Design review of the part built by this model. Coordinates are the model's own, in mm. Face numbers are marked on the shaded views. A direction names the side the tool comes from. Give positions to 0.01 mm unless a question says otherwise; leave off trailing zeros. Loops run counter-clockwise (first coordinate to the right, second up) from the corner with the lowest first, then second, coordinate; pieces in that order, holes last. Notation, with made-up numbers: (-27, 40) - (25, 40) arc R22 ccw to (25, 74) - close; hole circle Ø9 at (30.25, 62). An arc over 180 degrees is marked (long way). Write each question's results on one line, items separated by ' | '.
Autodesk Fusion 360 part; units mm, degrees
sketch "スケッチ1" plane through (0, 0, 0) normal (0, 0, 1) x (1, 0, 0)
  circle A0 centre (0, 0) radius 11
  dimension "d1" = 22
extrude "押し出し1" add sketch "スケッチ1" along normal blind 18
sketch "スケッチ2" plane through (0, 0, 18) normal (0, 0, 1) x (1, 0, 0)
  circle A0 centre (0, 0) radius 11
  circle A1 centre (0, 0) radius 10
  line L0 (-7, -7.7) -> (7, -7.7)
  line L1 (7, -7.7) -> (7, 7.7)
  line L2 (7, 7.7) -> (-7, 7.7)
  line L3 (-7, 7.7) -> (-7, -7.7)
  line L4 (-7, -7.7) -> (7, 7.7) construction
  line L5 (7, -7.7) -> (-7, 7.7) construction
  dimension "d4" = 20
  dimension "d5" = 14
  dimension "d6" = 15.4
sketch "スケッチ3" plane through (0, 0, 18) normal (0, 0, 1) x (1, 0, 0)
extrude "押し出し2" add sketch "スケッチ2" along normal blind 32 contours A1 L1 | A1 L0 L1 L2 L3 | A1 L3
sketch "スケッチ4" plane through (0, 0, 50) normal (0, 0, 1) x (1, 0, 0)
  arc A0 (6.3804, -7.7) -> (6.3804, 7.7) centre (0, 0) ccw
  line L0 (6.3804, 7.7) -> (-6.3804, 7.7)
  arc A1 (-6.3804, 7.7) -> (-6.3804, -7.7) centre (0, 0) ccw
  line L1 (-6.3804, -7.7) -> (6.3804, -7.7)
  circle A2 centre (0, 0) radius 10.2
  dimension "d9" = 20.4
extrude "押し出し3" add sketch "スケッチ4" along normal blind 9 contours A0 L0 A1 L1 | A2
sketch "スケッチ5" plane through (0, 0, 0) normal (0, 0, -1) x (-1, 0, 0)
  circle A0 centre (0, 0) radius 11
  circle A1 centre (0, 0) radius 6.9
  line L0 (6, 3.45) -> (-6, 3.45)
  line L1 (-6, 3.45) -> (-6, -3.45)
  line L2 (-6, -3.45) -> (6, -3.45)
  line L3 (6, -3.45) -> (6, 3.45)
  line L4 (6, 3.45) -> (-6, -3.45) construction
  line L5 (-6, 3.45) -> (6, -3.45) construction
  dimension "d12" = 13.8
  dimension "d13" = 12
  dimension "d14" = 6.9
extrude "押し出し4" add sketch "スケッチ5" along normal blind 2 contours A1 L3 | A1 L0 L1 L2 L3 | A1 L1
sketch "スケッチ6" plane through (0, 0, -2) normal (0, 0, -1) x (-1, 0, 0)
  arc A0 (-5.9756, 3.45) -> (-5.9756, -3.45) centre (0, 0) ccw
  line L0 (-5.9756, -3.45) -> (5.9756, -3.45)
  arc A1 (5.9756, -3.45) -> (5.9756, 3.45) centre (0, 0) ccw
  line L1 (5.9756, 3.45) -> (-5.9756, 3.45)
  circle A2 centre (0, 0) radius 2
  dimension "d17" = 4
extrude "押し出し5" add sketch "スケッチ6" along normal blind 4 contours A2
sketch "スケッチ8" plane through (0, 0, 18) normal (0, 0, 1) x (1, 0, 0)
  circle A0 centre (0, 0) radius 2
  dimension "d22" = 4
extrude "押し出し6" add 1 faces at (-0.637, 0.1965, -6) along direction (0, 0, -1) blind 8
sketch "スケッチ9" plane through (0, 0, -14) normal (0, 0, -1) x (-1, 0, 0)
  circle A0 centre (0, 0) radius 2
  line L0 (0, 2) -> (-2.3, 2)
  line L1 (-2.3, 2) -> (-2.3, 1.5)
  line L2 (-2.3, 1.5) -> (0, 1.5)
  line L3 (0, 1.5) -> (0, 2)
  circle A1 centre (0, 0) radius 2
  line L4 (0, 1.5) -> (1.7491, 1.5)
  line L5 (1.7491, 1.5) -> (1.7491, 2)
  line L6 (1.7491, 2) -> (0, 2)
  line L7 (0, 2) -> (0, 1.5)
extrude "押し出し7" cut sketch "スケッチ9" against normal blind 8 contours A0 L3 A1 L4 L7 | A0 L2 L3 A1 L7
sketch "スケッチ10" plane through (0, 0, 0) normal (0, 0, -1) x (-1, 0, 0)
  line L0 (-5.9756, 3.45) -> (5.9756, 3.45)
  arc A0 (5.9756, -3.45) -> (5.9756, 3.45) centre (0, 0) ccw
  line L1 (5.9756, -3.45) -> (-5.9756, -3.45)
  arc A1 (-5.9756, 3.45) -> (-5.9756, -3.45) centre (0, 0) ccw
  circle A2 centre (0, 0) radius 11
  circle A3 centre (0, 0) radius 7
  line L2 (7, 6) -> (-7, 6)
  line L3 (-7, 6) -> (-7, -6)
  line L4 (-7, -6) -> (7, -6)
  line L5 (7, -6) -> (7, 6)
  line L6 (7, 6) -> (-7, -6) construction
  line L7 (-7, 6) -> (7, -6) construction
  dimension "d27" = 14
  dimension "d28" = 14
  dimension "d29" = 12
extrude "押し出し8" add sketch "スケッチ10" along normal blind 2 contours A3 L2 L4
sketch "スケッチ11" plane through (0, 0, 0) normal (0, 0, -1) x (-1, 0, 0)
  line L0 (-3.6056, 6) -> (3.6056, 6)
  arc A0 (3.6056, -6) -> (3.6056, 6) centre (0, 0) ccw
  line L1 (3.6056, -6) -> (-3.6056, -6)
  arc A1 (-3.6056, 6) -> (-3.6056, -6) centre (0, 0) ccw
  circle A2 centre (0, 0) radius 11
sketch "スケッチ12" plane through (0, 0, 0) normal (0, 0, -1) x (-1, 0, 0)
  line L0 (11, 0) -> (-11, 0)
  line L1 (-11, 0) -> (-11, -11)
  line L2 (-11, -11) -> (0, 0)
  line L3 (0, 0) -> (7.7782, 7.7782)
  circle A0 centre (0, 0) radius 9
  circle A1 centre (-6.364, -6.364) radius 1
  line L4 (0, 1.75) -> (0, 22.5)
  circle A2 centre (6.364, -6.364) radius 1
  circle A3 centre (6.364, 6.364) radius 1
  circle A4 centre (-6.364, 6.364) radius 1
  dimension "d32" = 11
  dimension "d33" = 180
  dimension "d34" = 11
  dimension "d35" = 18
  dimension "d36" = 2
extrude "押し出し9" cut sketch "スケッチ12" against normal blind 4 contours L3 A0 A3 | L3 A0 A3 | A0 A2 | A0 A2 | L2 A0 A1 | L2 A0 A1 | L3 A0 A3 | L3 A0 A3 | A0 A4 | A0 A4 | L2 A0 A1 | L2 A0 A1
sketch "スケッチ14" plane through (0, 0, 50) normal (0, 0, -1) x (-1, 0, 0)
  circle A0 centre (0, 0) radius 10.2
  line L0 (6.3804, -7.7) -> (-6.3804, -7.7)
  arc A1 (-6.3804, 7.7) -> (-6.3804, -7.7) centre (0, 0) ccw
  line L1 (-6.3804, 7.7) -> (6.3804, 7.7)
  arc A2 (6.3804, -7.7) -> (6.3804, 7.7) centre (0, 0) ccw
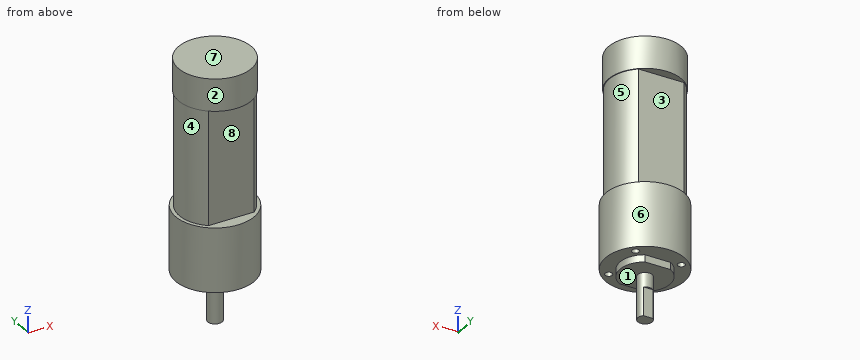
Item 1: We need section D-D on y = 4. Give the boundary of the cut face in (x, z), then the cut area to 3 significant figures.
Output values:
outline: (-10.25, 0) - (-5.74, 0) - (-5.74, -2) - (5.74, -2) - (5.74, 0) - (10.25, 0) - (10.25, 18) - (9.17, 18) - (9.17, 50) - (9.38, 50) - (9.38, 59) - (-9.38, 59) - (-9.38, 50) - (-9.17, 50) - (-9.17, 18) - (-10.25, 18) - close | area: 1,150 mm²
Item 2: Clearance check with flat-ended pins moving along their axes: P1, Ø6, axis at x = -2, y = 4, coming from the -Z side; P2, Ø0.6, axis at x = -1, z = -1.5, coming from the -Y side; P3, Ø1, axis at x = -7, y = -6.5, coming from the -Z side; P4, Ø10, axis at y = -8.5, z = 6.5, coming from the -X side. State where each tip first meets the part, or that it passes through.
Output values:
P1: stops at z = -14 | P2: stops at y = -6 | P3: stops at z = 0 | P4: stops at x = -10.43
Item 3: Tool access review of the marked faces 1, 2, 3 and 4: name each direction out of +Z, -Z, +X, -X, +Y, -Y from which nothing blocks a thin tool from reaching the whole face with its end or side.
Output values:
face 1: -Z | face 2: +Z | face 3: +X, -X, +Y | face 4: -X
Item 4: Draft analysis for pull direction Z (two halves, no side actions). For the marked faces 5, 6, 7 and 8, state which applies: +Z half, -Z half, draft (parallel to the pull), parting line (faces both ways), or undercut.
Output values:
face 5: undercut | face 6: draft | face 7: +Z half | face 8: undercut
Item 5: We need section A-A on x = 0. Give the boundary of the cut face in (y, z), then the cut area to 3 significant figures.
Output values:
outline: (-11, 0) - (-6, 0) - (-6, -2) - (-2, -2) - (-2, -14) - (1.5, -14) - (1.5, -6) - (2, -6) - (2, -2) - (6, -2) - (6, 0) - (11, 0) - (11, 18) - (7.7, 18) - (7.7, 50) - (10.2, 50) - (10.2, 59) - (-10.2, 59) - (-10.2, 50) - (-7.7, 50) - (-7.7, 18) - (-11, 18) - close | area: 1,140 mm²
Item 6: We need section C-C on y = 0. Give the boundary of the cut face in (x, z).
Output values:
outline: (-11, 0) - (-7, 0) - (-7, -2) - (-2, -2) - (-2, -14) - (2, -14) - (2, -2) - (7, -2) - (7, 0) - (11, 0) - (11, 18) - (10, 18) - (10, 50) - (10.2, 50) - (10.2, 59) - (-10.2, 59) - (-10.2, 50) - (-10, 50) - (-10, 18) - (-11, 18) - close
Item 7: Wall thickness on probe 1 along Z at (x, y) = (0.5, 10); probe 2 along Z at (x, y) = (2, 2.75); probe 3 along Z at (x, y) = (8.75, -6): over which ranges is each line inside the solid? List them lowest first.
Output values:
probe 1: z = 0 to 18, 50 to 59 | probe 2: z = -2 to 59 | probe 3: z = 0 to 18
Item 8: We need section B-B on z = 2. Give the boundary of the cut face in (x, y), then the cut area to 3 significant figures.
Output values:
outline: circle Ø22 at (0, 0); hole circle Ø2 at (-6.36, -6.36); hole circle Ø2 at (-6.36, 6.36); hole circle Ø2 at (6.36, -6.36); hole circle Ø2 at (6.36, 6.36) | area: 368 mm²
